from build123d import *

# Parameters (mm, degrees)
BOSS_EXTRUDE9_START = -5
BOSS_EXTRUDE9_DEPTH = 5
SKETCH10_W          = 100.017630752
SKETCH10_H          = 82.257490713
CUT_EXTRUDE5_DEPTH  = 5


# Read off the part's stored shape, not the designer's step: Boss-Extrude9
with BuildPart() as part:
    # Sketch3 → Revolve4 (revolve)
    with BuildSketch(Plane.XY, mode=Mode.PRIVATE) as revolve4_sk:
        Polygon((-45.345396491, 59.752657492), (-50.285549319, 51.471259135), (-37.687875269, 51.471259135), (-37.687875269, 71.31273478), (-45.345396491, 71.31273478), align=None)
    revolve(revolve4_sk.sketch.rotate(Axis((-37.687875269, 51.471259135, 0), (0, 1, 0)), 270), axis=Axis((-37.687875269, 51.471259135, 0), (0, 1, 0)))

    # Sketch5 → Revolve5 (revolve)
    with BuildSketch(Plane(origin=(0, 97.31273478, 0), x_dir=(1, 0, 0), z_dir=(0, 1, 0)), mode=Mode.PRIVATE) as revolve5_sk:
        Polygon((-37.687875269, 0), (-37.302956611, -20), (-65.802956611, -20), (-69.265253256, 29.40337608), (-38.265253256, 30), align=None)
    revolve(revolve5_sk.sketch.rotate(Axis((-37.687875269, 97.31273478, 0), (-0.01924236949216868, 0, -0.9998148484676185)), 180), axis=Axis((-37.687875269, 97.31273478, 0), (-0.01924236949216868, 0, -0.9998148484676185)))

    # Boss-Extrude9 outline → Boss-Extrude9 (add)
    with BuildSketch(Plane.XY.offset(-25).offset(BOSS_EXTRUDE9_START)):
        with BuildLine():
            ThreePointArc((-4.286962272, 87.31273478), (-2.827981935, 97.31273478), (-4.286962272, 107.31273478))
            Line((-4.286962272, 107.31273478), (-9.761081063, 107.31273478))
            Line((-9.761081063, 107.31273478), (-9.761081063, 87.31273478))
            Line((-9.761081063, 87.31273478), (-4.286962272, 87.31273478))
        make_face()
        with BuildLine():
            ThreePointArc((-66.708431797, 87.31273478), (-68.390710613, 97.31273478), (-66.708431797, 107.31273478))
            Line((-66.708431797, 107.31273478), (-71.369001597, 107.31273478))
            ThreePointArc((-71.369001597, 107.31273478), (-72.827981935, 97.31273478), (-71.369001597, 87.31273478))
            Line((-71.369001597, 87.31273478), (-66.708431797, 87.31273478))
        make_face()
    extrude(amount=BOSS_EXTRUDE9_DEPTH)

    # Sketch10 → Cut-Extrude5 (cut)
    with BuildSketch(Plane.XY.offset(-29.00378798)):
        with Locations((-35.882792004, 102.435950212)):
            Rectangle(SKETCH10_W, SKETCH10_H)
    extrude(amount=-CUT_EXTRUDE5_DEPTH, mode=Mode.SUBTRACT)

    # Sketch6 → Cut-Revolve4 (revolve, cut)
    with BuildSketch(Plane(origin=(0, 97.31273478, 0), x_dir=(1, 0, 0), z_dir=(0, 1, 0))):
        Polygon((-37.370304904, -16.50064803), (-62.508760096, -16.940904481), (-65.765253256, 30.531390366), (-38.285658965, 31.060260794), align=None)
    revolve(axis=Axis((-38.285658965, 97.31273478, -31.060260794), (0.019242369492168804, 0, 0.9998148484676185)), mode=Mode.SUBTRACT)


solid = part.part
Design review of the part built by this model. Coordinates are the model's own, in mm. A direction names the side the tool comes from. Round coordinates to 2 decimals unless told otherwise and drop trailing zeros. One line per item, written item: value. Start each with the question number.
1) To check wall thickness, follow L1, parallel to Y at x = -48.5, z = 2.5; L2, parallel to Y at x = -29, z = -1.5; L3, parallel to X at y = 113, z = -9. State the ranges of each line that lie inside material, in increasing order. Write a range as from..to.
2) Consider section A-A on z = -11.5. Give the number of separate pieces and of enclosed holes in the cut face, then the cut area to 3 significant figures.
3) Insertion check: pin 1 Ø2 at (x, z) = (-6.5, -27.5) entering from -Y; pin 2 Ø8 at (y, z) = (70, 15) entering from -X; pin 3 Ø3 at (x, z) = (-69.5, -27.5) entering from +Y. Each pin has a flat end and moves straight along its axis. Give the tip position at first contact, or say it passes through.
4) For faces 1 (the conical face through (-37.03, 98.85, 16.49)), 2 (the cylindrical face through (-33.03, 64.26, 6.08)), 3 (the conical face through (-39, 97, 20)), list the 3-axis set-ups (+Z, -Z, +X, -X, +Y, -Y) from which the entire face can be reached by the end or side of a thin tool; tool diameter is ignored.
5) Draft analysis for pull direction Y (two halves, no side actions). For faces 4 (the flat face through (-69, 107.313, -27)), 5 (the conical face through (-34.398, 71.245, -6.925)), 6 (the cylindrical face through (-72.828, 97.455, -27.03)), state which applies: +Y half, -Y half, draft (parallel to the pull), parting line (faces both ways), or undercut.
Reported:
1. L1: y = 51.47..53.99, 70.03..73.86, 120.76..124.6
1. L2: y = 51.47..57.81, 69.08..72.8, 121.83..125.55
1. L3: x = -63.4..-59.12, -16.65..-12.39
2. separate pieces: 2
2. enclosed holes: 1
2. area: 643 mm^2
3. pin 1: stops at y = 87.31
3. pin 2: stops at x = -54.22
3. pin 3: stops at y = 107.31
4. face 1: -Z
4. face 2: none
4. face 3: +Z, +X
5. face 4: +Y half
5. face 5: undercut
5. face 6: parting line
